from build123d import *

# Parameters (mm, degrees)
F1_DEPTH = 3
F2_DEPTH = 3


with BuildPart() as f1:
    # F0 (on Top) → F1 (new body)
    with BuildSketch(Plane.XY):
        with BuildLine():
            ThreePointArc((0, 44.3587770077), (-50, 149.4337567297), (-100, 44.3587770077))
            Line((-100, 44.3587770077), (-100, 0))
            Line((-100, 0), (0, 0))
            Line((0, 0), (0, 44.3587770077))
        make_face()
        with BuildLine():
            ThreePointArc((-97, 46.1631766902), (-50, 145.9696551146), (-3, 46.1631766902))
            Line((-3, 46.1631766902), (-3, 3))
            Line((-3, 3), (-97, 3))
            Line((-97, 3), (-97, 46.1631766902))
        make_face(mode=Mode.SUBTRACT)
        with BuildLine():
            Line((-3, 3), (-3, 46.1631766902))
            ThreePointArc((-3, 46.1631766902), (-50, 145.9696551146), (-97, 46.1631766902))
            Line((-97, 46.1631766902), (-97, 3))
            Line((-97, 3), (-3, 3))
        make_face()
    extrude(amount=F1_DEPTH)

    # F0 (on Top) → F2 (join)
    with BuildSketch(Plane.XY):
        with BuildLine():
            Line((-3, 3), (-3, 46.1631766902))
            ThreePointArc((-3, 46.1631766902), (-50, 145.9696551146), (-97, 46.1631766902))
            Line((-97, 46.1631766902), (-97, 3))
            Line((-97, 3), (-3, 3))
        make_face()
    extrude(amount=-F2_DEPTH)


solid = f1.part
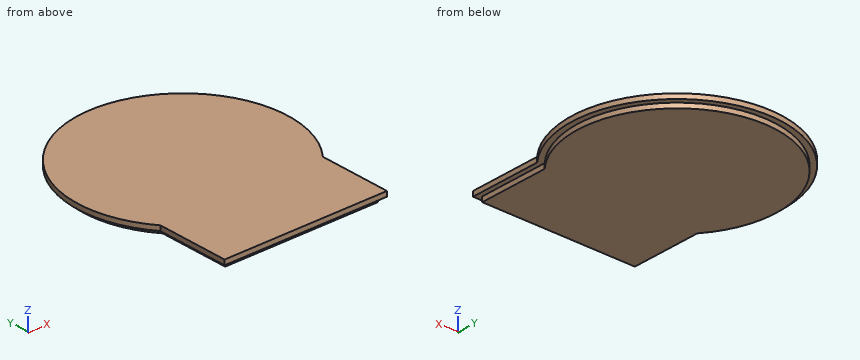
The model under review builds one solid part; all positions refer to its coordinate system, in mm. Give positions to 0.01 mm unless a question says otherwise; leave off trailing zeros. Loops run counter-clockwise (first coordinate to the right, second up) from the corner with the lowest first, then second, coordinate; pieces in that order, holes last. Notation, with made-up numbers: (62, -22) -> (117, -22) arc R18 ccw to (117, -13) -> close; hole circle Ø11 at (51, -38.75). An arc over 180 degrees is marked (long way). Put each result on its own line as item: value. Start each with the question number.
1. Clearance check with flat-ended pins moving along their axes: P1, Ø1, axis at y = 23, z = -2, coming from the +X side; P2, Ø2.5, axis at y = 19.5, z = 1, coming from the +X side; P3, Ø1.5, axis at x = -63.5, z = -2, coming from the -Y side. State where each tip first meets the part, or that it passes through.
2. We need section B-B on y = 35. State the section outline as (x, z) points.
3. We need section C-C on z = 1.75. State the section outline as (x, y) points, then the cut area to 3 significant figures.
4. We need section A-A on x = -50. State the section outline as (y, z) points.
5. Wall thickness on probe 1 along Z at (x, y) = (-3, 128); probe 2 along X at (y, z) = (36.5, 2.4); probe 3 along Y at (x, z) = (-3, 0.25): over which ranges is each line inside the solid? List them lowest first.
Determined:
1. P1: x = -3
1. P2: x = 0
1. P3: y = 3
2. outline: (-100, 0) -> (-97, 0) -> (-97, -3) -> (-3, -3) -> (-3, 0) -> (0, 0) -> (0, 3) -> (-100, 3) -> close
3. outline: (-100, 0) -> (0, 0) -> (0, 44.36) arc R64.43 ccw (long way) to (-100, 44.36) -> close
3. area: 15,800 mm^2
4. outline: (0, 0) -> (3, 0) -> (3, -3) -> (145.97, -3) -> (145.97, 0) -> (149.43, 0) -> (149.43, 3) -> (0, 3) -> close
5. probe 1: 0 to 3
5. probe 2: -100 to 0
5. probe 3: 0 to 129.08
